Can you work these out from the model? Positions are in its coordinate system, mm. A direction names the side the tool comes from. Give positions to 0.01 mm unless a question says otherwise; leave off trailing zeros. Write each loop counter-clockwise with the first axis right and the second up, starting at its lowest first coordinate (ties: lowest second). Pieces come first, ordered by that corner, then holes.
from build123d import *

# Parameters (mm, degrees)
SKETCH1_W           = 206.502
SKETCH1_H           = 34.9758
SKETCH1_R           = 1.4732
BOSS_EXTRUDE1_DEPTH = 5.4102


with BuildPart() as part:
    # Sketch1 → Boss-Extrude1 (new body)
    with BuildSketch(Plane.XY):
        Polygon((61.191000046, 23.8379), (61.191000046, 30.226), (-109.601, 30.226), (-109.601, 23.8379), (-128.27, 23.8379), (-128.27, -23.8379), (-109.601, -23.8379), (-109.601, -30.226), (61.191000046, -30.226), (61.191000046, -23.8379), (128.27, -23.8379), (128.27, 23.8379), align=None)
        Rectangle(SKETCH1_W, SKETCH1_H, mode=Mode.SUBTRACT)
        with Locations((-115.57, 17.4879)):
            Circle(SKETCH1_R, mode=Mode.SUBTRACT)
        with Locations((-115.57, -17.4879)):
            Circle(SKETCH1_R, mode=Mode.SUBTRACT)
        with Locations((115.57, -17.4879)):
            Circle(SKETCH1_R, mode=Mode.SUBTRACT)
        with Locations((115.57, 17.4879)):
            Circle(SKETCH1_R, mode=Mode.SUBTRACT)
    extrude(amount=BOSS_EXTRUDE1_DEPTH)


solid = part.part
(1) Will these pins go through, and if not, where does the flat tip stop? P1, Ø1.6, axis at x = 79.5, z = 2, coming from the -Y side; P2, Ø6, axis at x = 39.5, y = -12, coming from the +Z side; P3, Ø2.5, axis at x = -122, z = 3.5, coming from the +Y side.
Returned:
P1: stops at y = -23.84
P2: passes through
P3: stops at y = 23.84
(2) Imagine slicing it at A-A, the plane x = -78.5. Write out the boundary of the cut face in (y, z).
Returned:
outline: (-30.23, 0) - (-17.49, 0) - (-17.49, 5.41) - (-30.23, 5.41) - close; (17.49, 0) - (30.23, 0) - (30.23, 5.41) - (17.49, 5.41) - close
(3) Imagine slicing it at D-D, the plane x = 109. Write out the boundary of the cut face in (y, z).
Returned:
outline: (-23.84, 0) - (23.84, 0) - (23.84, 5.41) - (-23.84, 5.41) - close
(4) Imagine slicing it at C-C, the plane z = 3.7. Write out the boundary of the cut face in (x, y).
Returned:
outline: (-128.27, -23.84) - (-109.6, -23.84) - (-109.6, -30.23) - (61.19, -30.23) - (61.19, -23.84) - (128.27, -23.84) - (128.27, 23.84) - (61.19, 23.84) - (61.19, 30.23) - (-109.6, 30.23) - (-109.6, 23.84) - (-128.27, 23.84) - close; hole circle Ø2.95 at (-115.57, -17.49); hole circle Ø2.95 at (-115.57, 17.49); hole (-103.25, -17.49) - (103.25, -17.49) - (103.25, 17.49) - (-103.25, 17.49) - close; hole circle Ø2.95 at (115.57, -17.49); hole circle Ø2.95 at (115.57, 17.49)
(5) If I drill on L1, parallel to Y at x = -115.5, z = 0.6; L2, parallel to Y at x = -70, z = 2.05; L3, parallel to X at y = -11.5, z = 2.35, over which ranges is the centre line in solid material (lowest first)?
Returned:
L1: y = -23.84 to -18.96, -16.02 to 16.02, 18.96 to 23.84
L2: y = -30.23 to -17.49, 17.49 to 30.23
L3: x = -128.27 to -103.25, 103.25 to 128.27
(6) For faces 1 (the face through (61.191, 27, 3)), 2 (the face through (-119, 23.838, 3)), 3 (the face through (61.191, -27, 3)), which set-ups out of +Z, -Z, +X, -X, +Y, -Y let a thin tool reach every point of the face, with its end or its side?
Returned:
face 1: +Z, -Z, +X, +Y
face 2: +Z, -Z, -X, +Y
face 3: +Z, -Z, +X, -Y
(7) Imagine slicing it at B-B, the plane y = -3. Write out the boundary of the cut face in (x, z), plus the area to 3 significant figures.
Returned:
outline: (-128.27, 0) - (-103.25, 0) - (-103.25, 5.41) - (-128.27, 5.41) - close; (103.25, 0) - (128.27, 0) - (128.27, 5.41) - (103.25, 5.41) - close
area: 271 mm2
(8) If we mould it in two halves opening along Y, with no side actions, what happens to faces 4 (the face through (94, -23.838, 3)), 5 (the face through (-103.251, 0, 3)), 6 (the face through (-109.601, -27, 3)), 7 (the face through (-1, -17.488, 3))? For each: +Y half, -Y half, draft (parallel to the pull), parting line (faces both ways), or undercut.
Returned:
face 4: -Y half
face 5: undercut
face 6: draft
face 7: undercut
